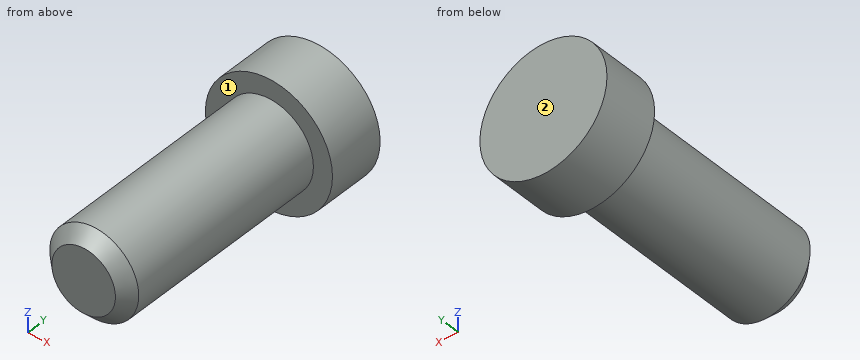
```python
from build123d import *

# Parameters (mm, degrees)
F0_R     = 4.445
F1_DEPTH = 22.225
F2_R     = 6.35
F2_R_2   = 4.445
F3_DEPTH = 5.715
F4_SIZE  = 1.27


with BuildPart() as f1:
    # F0 (on Front) → F1 (new body)
    with BuildSketch(Plane.XZ):
        Circle(F0_R)
    extrude(amount=F1_DEPTH)

    # F2 (on face) → F3 (join)
    with BuildSketch(Plane(origin=(0, 0, 0), x_dir=(-1, 0, 0), z_dir=(0, 1, 0))):
        Circle(F2_R)
        Circle(F2_R_2, mode=Mode.SUBTRACT)
        Circle(F2_R_2)
    extrude(amount=F3_DEPTH)

    # F4
    f4_edges = [f1.edges().sort_by_distance(p)[0] for p in [
        (-4.445, -22.225, 0),
    ]]
    chamfer(f4_edges, length=F4_SIZE)


solid = f1.part
```
Verification items for the finished model (mm, model axes). Face numbers are marked on the shaded views. A direction names the side the tool comes from. Coordinates: 2 decimals unless noted, no trailing zeros. Write each loop counter-clockwise with the first axis right and the second up, starting at its lowest first coordinate (ties: lowest second). Pieces come first, ordered by that corner, then holes. Notation, with made-up numbers: M -28.5,-31 L 30.5,-31 A20 cw 30.5,-20 Z; hole C 27.25,13 d11. An arc over 180 degrees is marked long. Answer as a JSON object with one key per item and string values. Group by question number.
(1) Cross-section at C-C, the plane y = 0.75. Record the cut outline in (x, z).
(2) Gauge pin test, flat ends, axial feed: pin 1 (6 mm diameter, centred on y = -7.5, z = -2.5, fed in from +X) (3 decimals); pin 2 (1.5 mm diameter, centred on x = 2.5, y = -12.5, fed in from -Z); pin 3 (3 mm diameter, centred on x = 3.5, y = -7.5, fed in from -Z). Record the tip position at first contact, or that the pin passes through.
(3) Material ranges on line 1 (Y direction, x = -0.25, z = -6) (3 decimals); line 2 (X direction, y = 1.5, z = -0.25); line 3 (X direction, y = 4, z = 1.75), recorded low to high.
(4) Tool access check on the marked faces 1 and 2. Record the directions out of +Z, -Z, +X, -X, +Y, -Y that give a thin tool (end or side, any length) a straight path to the whole face; none if there is none.
(5) Cross-section at B-B, the plane z = 0. Record the cut outline in (x, y) (3 decimals).
(6) Cross-section at D-D, the plane z = -5. Record the cut outline in (x, y) (3 decimals).
(7) Cross-section at A-A, the plane x = 0. Record the cut outline in (y, z) (3 decimals), and give its area (3 significant figures).
Reply:
{
 "1": {"outline": "C 0,0 d12.7"},
 "2": {"pin 1": "x = 4.445", "pin 2": "z = -4.09", "pin 3": "z = -3.97"},
 "3": {"line 1": "0 to 5.715", "line 2": "-6.35 to 6.35", "line 3": "-6.1 to 6.1"},
 "4": {"face 1": "-Y", "face 2": "+Z, -Z, +X, -X, +Y"},
 "5": {"outline": "M -6.35,0 L -4.445,0 L -4.445,-20.955 L -3.175,-22.225 L 3.175,-22.225 L 4.445,-20.955 L 4.445,0 L 6.35,0 L 6.35,5.715 L -6.35,5.715 Z"},
 "6": {"outline": "M -3.914,0 L 3.914,0 L 3.914,5.715 L -3.914,5.715 Z"},
 "7": {"outline": "M -22.225,-3.175 L -20.955,-4.445 L 0,-4.445 L 0,-6.35 L 5.715,-6.35 L 5.715,6.35 L 0,6.35 L 0,4.445 L -20.955,4.445 L -22.225,3.175 Z", "area": "269 mm²"}
}
